from build123d import *

# Parameters (mm, degrees)
SKETCH_1_W      = 228
SKETCH_1_H      = 84
SKETCH_1_R      = 1.6
SKETCH_1_R_2    = 2.15
EXTRUDE_1_DEPTH = 1


with BuildPart() as part:
    # Эскиз1 → Вытянуть1 (new body)
    with BuildSketch(Plane.XY):
        Rectangle(SKETCH_1_W, SKETCH_1_H)
        with Locations((23.5, -2)):
            Circle(SKETCH_1_R, mode=Mode.SUBTRACT)
        with Locations((107, 32)):
            Circle(SKETCH_1_R_2, mode=Mode.SUBTRACT)
        with Locations(Location((-107, 32, 0), (0, 0, 180))):
            Circle(SKETCH_1_R_2, mode=Mode.SUBTRACT)
        with Locations((-107, -32)):
            Circle(SKETCH_1_R_2, mode=Mode.SUBTRACT)
        with Locations(Location((107, -32, 0), (0, 0, 180))):
            Circle(SKETCH_1_R_2, mode=Mode.SUBTRACT)
        with Locations((88.5, -2)):
            Circle(SKETCH_1_R, mode=Mode.SUBTRACT)
        with BuildLine():
            Line((41, 3.5), (71, 3.5))
            ThreePointArc((71, 3.5), (78.5, -4), (71, -11.5))
            Line((71, -11.5), (41, -11.5))
            ThreePointArc((41, -11.5), (33.5, -4), (41, 3.5))
        make_face(mode=Mode.SUBTRACT)
    extrude(amount=EXTRUDE_1_DEPTH)


solid = part.part
The listing builds one solid part. Answer for the finished solid, in the listing's coordinates (mm). A direction names the side the tool comes from. Give positions to 0.01 mm unless a question says otherwise; leave off trailing zeros. Loops run counter-clockwise (first coordinate to the right, second up) from the corner with the lowest first, then second, coordinate; pieces in that order, holes last. Notation, with made-up numbers: M -4,-12 L 45,-12 A16 cw 45,-8 Z; hole C 38,66.25 d1. An arc over 180 degrees is marked long. Answer as CSV lines item,"result".
Item 1: Which of the six approach directions +Z, -Z, +X, -X, +Y, -Y give full straight-line access (tool end or side, diameter ignored) to faces 3 (the cylindrical face through (78.5, -3.84, 0.49)), 4 (the flat face through (-2, 1, 1))?
Values follow:
face 3,"+Z, -Z"
face 4,"+Z, +X, -X, +Y, -Y"
Item 2: The part is cut by section B-B (y = 32). Give the vertices of the cut face in (x, z).
Values follow:
outline,"M -114,0 L -109.15,0 L -109.15,1 L -114,1 Z; M -104.85,0 L 104.85,0 L 104.85,1 L -104.85,1 Z; M 109.15,0 L 114,0 L 114,1 L 109.15,1 Z"
Item 3: The part is cut by section A-A (x = 55). Give the vertices of the cut face in (y, z).
Values follow:
outline,"M -42,0 L -11.5,0 L -11.5,1 L -42,1 Z; M 3.5,0 L 42,0 L 42,1 L 3.5,1 Z"
Item 4: Given pin 1 Ø3.5 at (x, y) = (107, -32) entering from -Z, flat-ended and moving along its own axis, determine where the tip first touches the part or whether it passes through.
Values follow:
pin 1,"passes through"
Item 5: The mould has two halves that part along Y. Classify faces 1 (the cylindrical face through (105.415, 33.453, 0.493)), 2 (the flat face through (-2, 1, 0)): released by +Y, released by -Y, zero draft, split by the parting line, or undercut.
Values follow:
face 1,"undercut"
face 2,"zero draft"
Item 6: The part is cut by section D-D (x = 107). Give the vertices of the cut face in (y, z).
Values follow:
outline,"M -42,0 L -34.15,0 L -34.15,1 L -42,1 Z; M -29.85,0 L 29.85,0 L 29.85,1 L -29.85,1 Z; M 34.15,0 L 42,0 L 42,1 L 34.15,1 Z"
Item 7: The part is cut by section C-C (z = 0.65). Give the vertices of the cut face in (x, y).
Values follow:
outline,"M -114,-42 L 114,-42 L 114,42 L -114,42 Z; hole C -107,-32 d4.3; hole C -107,32 d4.3; hole C 23.5,-2 d3.2; hole M 41,-11.5 L 71,-11.5 A7.5 ccw 71,3.5 L 41,3.5 A7.5 ccw Z; hole C 88.5,-2 d3.2; hole C 107,-32 d4.3; hole C 107,32 d4.3"
Item 8: Straight lines are drawn through the part: line 1 along Y through (x, z) = (-107, 0.55); line 2 along Y through (x, z) = (88.5, 0.8); line 3 along X through (y, z) = (-4, 0.3). For each, find the intervals that lie inside material, in ascending order. Write a range as [from, to].
Values follow:
line 1,"y = [-42, -34.15], [-29.85, 29.85], [34.15, 42]"
line 2,"y = [-42, -3.6], [-0.4, 42]"
line 3,"x = [-114, 33.5], [78.5, 114]"
